CAD build for the part. Positions are in the model's coordinates, mm. A direction names the side the tool comes from. Round coordinates to 2 decimals unless told otherwise and drop trailing zeros. Order: outer loops, then holes, each group sorted by start corner. A loop starts at its lowest first (then second) coordinate and runs counter-clockwise, first axis right, second up. Notation, with made-up numbers: M 1.25,-23 L 38.25,-23 A9 ccw 38.25,-13 Z; hole C 25,81 d6. An arc over 180 degrees is marked long. Put each result on its own line as item: value.
```python
from build123d import *

# Parameters (mm, degrees)
IZIM2_W           = 24.151632934
IZIM2_H           = 17.006179403
KES_D_ND_R1_ANGLE = 180


with BuildPart() as part:
    # Çizim1 → Döndür1 (revolve)
    with BuildSketch(Plane.XY):
        Polygon((0, 29.195939483), (-35.343100252, 29.195939483), (-35.343100252, 58.1627654), (-20.19122208, 58.1627654), (-20.19122208, 38.777274209), (0, 38.777274209), align=None)
    revolve(axis=Axis((0, 0, 0), (-1, 0, 0)))

    # Çizim2 → Kes-Döndür1 (revolve, symmetric, cut)
    with BuildSketch(Plane.XY) as kes_d_nd_r1_sk:
        with Locations((-20.013486139, 58.073305733)):
            Rectangle(IZIM2_W, IZIM2_H)
    revolve(axis=Axis((0, 0, 0), (-1, 0, 0)), revolution_arc=KES_D_ND_R1_ANGLE / 2, mode=Mode.SUBTRACT)
    revolve(kes_d_nd_r1_sk.sketch, axis=Axis((0, 0, 0), (1, 0, 0)), revolution_arc=KES_D_ND_R1_ANGLE / 2, mode=Mode.SUBTRACT)


solid = part.part
```
Item 1: Probe line 1 along Y through (x, z) = (-10.5, 0); line 2 along Y through (x, z) = (-23, 0). List the from-to ranges inside material, lowest first. Write a range as [from, to].
Answers below:
line 1: [-38.78, -29.2], [29.2, 38.78]
line 2: [-58.16, -29.2], [29.2, 49.57]
Item 2: Mould opens along Y. For faces 5 (the flat face through (-20.191, -40, 4)), 6 (the cylindrical face through (-17.919, 15.696, -24.618)), 7 (the cylindrical face through (-10, 37, -11.6)) say: pulls with the +Y half, pulls with the -Y half, needs draft (parallel to the pull), parting line crosses it, or undercut.
Answers below:
face 5: needs draft
face 6: undercut
face 7: parting line crosses it
Item 3: Band-saw the part on B-B on x = -24.5. Give the cut face in (y, z), and give its area (3 significant figures).
Answers below:
outline: M 0,-58.16 L 0,-49.57 A49.57 ccw 0,49.57 L 0,58.16 A58.16 ccw Z; hole C 0,0 d58.39
area: 6,500 mm²
Item 4: Band-saw the part on C-C on y = -13.5. Give the cut face in (x, z).
Answers below:
outline: M -35.34,-56.57 L -20.19,-56.57 L -20.19,-36.35 L 0,-36.35 L 0,-25.89 L -35.34,-25.89 Z; M -35.34,25.89 L 0,25.89 L 0,36.35 L -20.19,36.35 L -20.19,56.57 L -35.34,56.57 Z
Item 5: Tool access for faces 1 (the cylindrical face through (-26.06, 49.56, 1.09)), 2 (the flat face through (-26, 0, 54)), 3 (the flat face through (-26, 0, -54)), 4 (the flat face through (0, 6, -29)): list every direction of +Z, -Z, +X, -X, +Y, -Y with a clear straight run to the whole face (end or side of a thin tool).
Answers below:
face 1: +X, +Y
face 2: +Z, +X, +Y
face 3: -Z, +X, +Y
face 4: +Z, -Z, +X, +Y, -Y
Item 6: Pin check, flat tips, straight feed: P1, Ø5, axis at x = -25, z = -33, coming from the +Y side; P2, Ø5, axis at x = -27, y = 15.5, coming from the +Z side; P3, Ø2.5, axis at x = -24.5, z = -53.5, coming from the +Y side; P4, Ø12, axis at x = -7.5, z = 46.5, coming from the +Y side. Stop position of each tip, or through.
Answers below:
P1: y = 39.08
P2: z = 47.84
P3: y = 0
P4: through
Item 7: Band-saw the part on A-A on z = 0. Give the cut face in (x, y).
Answers below:
outline: M -35.34,-58.16 L -20.19,-58.16 L -20.19,-38.78 L 0,-38.78 L 0,-29.2 L -35.34,-29.2 Z; M -35.34,29.2 L 0,29.2 L 0,38.78 L -20.19,38.78 L -20.19,49.57 L -32.09,49.57 L -32.09,58.16 L -35.34,58.16 Z
Item 8: Band-saw the part on D-D on z = 18. Give the cut face in (x, y), and give its area (3 significant figures).
Answers below:
outline: M -35.34,-55.31 L -20.19,-55.31 L -20.19,-34.35 L 0,-34.35 L 0,-22.99 L -35.34,-22.99 Z; M -35.34,22.99 L 0,22.99 L 0,34.35 L -20.19,34.35 L -20.19,46.19 L -32.09,46.19 L -32.09,55.31 L -35.34,55.31 Z
area: 1,330 mm²
